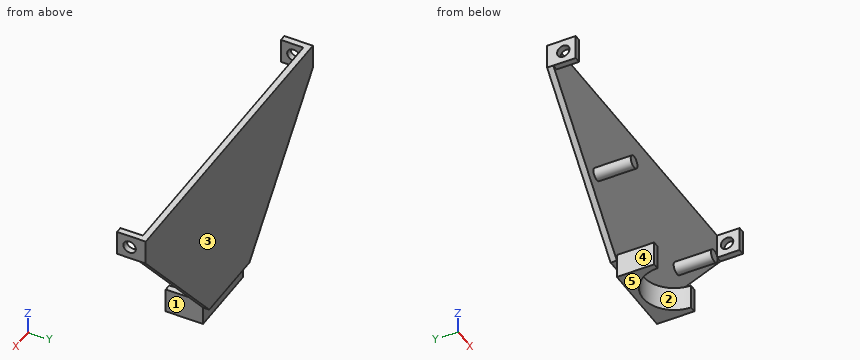
Solid Edge part; units mm, degrees
sketch "Sketch1" plane through (0, 0, 0) normal (0, -1, 0) x (1, 0, 0)
  line L0 (110.6916, 92.473) -> (110.6916, 112.473)
  line L1 (110.6916, 112.473) -> (-139.3084, 112.473)
  line L2 (-139.3084, 112.473) -> (-139.3084, 92.473)
  line L3 (-139.3084, 92.473) -> (-44.3084, -17.527)
  line L4 (-44.3084, -17.527) -> (15.6916, -17.527)
  line L5 (15.6916, -17.527) -> (110.6916, 92.473)
  dimension "D1" = 139.3084
  dimension "D2" = 110.6916
  dimension "D3" = 44.3084
  dimension "D4" = 110.6916
extrude "ExtrudedProtrusion_1" add sketch "Sketch1" against normal blind 5
sketch "Sketch2" plane through (10.6916, 0, 44.973) normal (0, -1, 0) x (1, 0, 0)
  line L0 (95, 47.5) -> (100, 47.5)
  line L1 (100, 47.5) -> (100, 67.5)
  line L2 (100, 67.5) -> (95, 67.5)
  line L3 (95, 67.5) -> (95, 47.5)
  line L4 (-55, -77.5) -> (5, -77.5)
  line L5 (5, -77.5) -> (5, -57.5)
  line L6 (5, -57.5) -> (-55, -57.5)
  line L7 (-55, -57.5) -> (-55, -77.5)
  circle A0 centre (-85, -5.5) radius 5
  circle A1 centre (35, -5.5) radius 5
  line L8 (-150, 47.5) -> (-145, 47.5)
  line L9 (-145, 47.5) -> (-145, 67.5)
  line L10 (-145, 67.5) -> (-150, 67.5)
  line L11 (-150, 67.5) -> (-150, 47.5)
  dimension "D1" = 150
  dimension "D2" = 145
  dimension "D3" = 145
  dimension "D4" = 100
  dimension "D5" = 95
  dimension "D6" = 55
  dimension "D7" = 55
extrude "Protrusion1" add sketch "Sketch2" along normal blind 30
sketch "Sketch3" plane through (-14.3084, -50, 24.202) normal (0, 0, 1) x (0, 1, 0)
  circle A0 centre (20, 0) radius 25
extrude "Cutout1" cut sketch "Sketch3" against normal through all
sketch "Sketch4" plane through (110.6916, -12.5, 102.473) normal (1, 0, 0) x (0, 1, 0)
  line L0 (-19.8844, -11.6156) -> (-5.5406, -11.6156)
  line L1 (-5.5406, -11.6156) -> (-5.5406, 11.1656)
  line L2 (-5.5406, 11.1656) -> (-19.8844, 11.1656)
  line L3 (-19.8844, 11.1656) -> (-19.8844, -11.6156)
  circle A0 centre (4.5, 0) radius 5
  dimension "D1" = 4.5
extrude "ExtrudedCutout_3" cut sketch "Sketch4" against normal blind 287.5314
Read the model definition and answer for the solid it produces. Units are mm, in the model's axes. Face numbers are marked on the shaded views. A direction names the side the tool comes from. Give positions to 0.01 mm unless a question says otherwise; leave off trailing zeros. Loops run counter-clockwise (first coordinate to the right, second up) from the corner with the lowest first, then second, coordinate; pieces in that order, holes last.
Item 1: For the marked faces 4 and 5, determine the directions among +Z, -Z, +X, -X, +Y, -Y from which every point of the face is accessible in a straight line to the end or side of a thin tool.
Item 2: Find the intervals of material crossed by line 1 along Z through (x, y) = (109.3, -8); line 2 along Y through (x, z) = (30.5, 104.5); line 3 along X through (y, z) = (-13, 42), in increasing order.
Item 3: The part is cut by section C-C (y = -22). Write down the section's boundary in (x, z).
Item 4: The part is cut by section A-A (y = -8). Write down the section's boundary in (x, z).
Item 5: The part is cut by section D-D (z = 63). Write down the section's boundary in (x, y).
Item 6: The part is cut by section B-B (x = -35). Write down the section's boundary in (y, z).
Item 7: The mould has two halves that part along X. Classify the marked faces 1, 2 and 3: released by +X, released by -X, zero draft, split by the parting line, or undercut.
Item 8: Each of these flat-tipped pins is pushed along its axis until it touches: pin 1 Ø6 at (x, y) = (-64.5, -17) entering from -Z; pin 2 Ø2.5 at (x, z) = (108.5, 98) entering from -Y; pin 3 Ø4 at (x, y) = (47, -2.5) entering from +Z; pin 4 Ø9 at (x, y) = (-29, -10.5) entering from +Z. Where does it stop, or does it pass through?
Taken from the geometry:
1. face 4: +Z, -Z, -X, -Y
1. face 5: -Z, +X, -X, +Y, -Y
2. line 1: z = 92.47 to 97.47, 107.47 to 112.47
2. line 2: y = 0 to 5
2. line 3: x = -78.62 to -69.99, 41.38 to 50.01
3. outline: circle Ø10 at (-74.31, 39.47); (-44.31, -32.53) - (-37.99, -32.53) - (-37.99, -12.53) - (-44.31, -12.53) - close; (9.38, -32.53) - (15.69, -32.53) - (15.69, -12.53) - (9.38, -12.53) - close; circle Ø10 at (45.69, 39.47)
4. outline: (-139.31, 92.47) - (-134.31, 92.47) - (-134.31, 97.47) - (-139.31, 97.47) - close; (-139.31, 107.47) - (-134.31, 107.47) - (-134.31, 112.47) - (-139.31, 112.47) - close; circle Ø10 at (-74.31, 39.47); (-44.31, -32.53) - (-26.18, -32.53) - (-26.18, -12.53) - (-44.31, -12.53) - close; (-2.43, -32.53) - (15.69, -32.53) - (15.69, -12.53) - (-2.43, -12.53) - close; circle Ø10 at (45.69, 39.47); (105.69, 92.47) - (110.69, 92.47) - (110.69, 97.47) - (105.69, 97.47) - close; (105.69, 107.47) - (110.69, 107.47) - (110.69, 112.47) - (105.69, 112.47) - close
5. outline: (-113.85, 0) - (85.24, 0) - (85.24, 5) - (-113.85, 5) - close
6. outline: (-15.97, -32.53) - (0, -32.53) - (0, -17.53) - (5, -17.53) - (5, 112.47) - (0, 112.47) - (0, -12.53) - (-15.97, -12.53) - close
7. face 1: released by +X
7. face 2: undercut
7. face 3: zero draft
8. pin 1: passes through
8. pin 2: stops at y = -18.04
8. pin 3: stops at z = 44.47
8. pin 4: stops at z = -12.53
